```python
from build123d import *

# Parameters (mm, degrees)
BOSS_EXTRUDE1_DEPTH = 10
SKETCH2_W           = 90
SKETCH2_H           = 10
BOSS_EXTRUDE2_DEPTH = 13
SKETCH3_W           = 90
SKETCH3_H           = 10
BOSS_EXTRUDE3_DEPTH = 13
SKETCH4_R           = 3
CUT_EXTRUDE2_DEPTH  = 13


with BuildPart() as part:
    # Sketch1 → Boss-Extrude1 (new, symmetric)
    with BuildSketch(Plane.XY):
        Polygon((-49.027757444, 0), (100.972242556, 0), (-49.027757444, 13.123299529), align=None)
    extrude(amount=BOSS_EXTRUDE1_DEPTH, both=True)

    # Sketch2 → Boss-Extrude2 (add)
    with BuildSketch(Plane.XY.offset(10)):
        with Locations((30.972242556, 5)):
            Rectangle(SKETCH2_W, SKETCH2_H)
    extrude(amount=BOSS_EXTRUDE2_DEPTH)

    # Sketch3 → Boss-Extrude3 (add)
    with BuildSketch(Plane.XY.offset(-10)):
        with Locations((30.972242556, 5)):
            Rectangle(SKETCH3_W, SKETCH3_H)
    extrude(amount=-BOSS_EXTRUDE3_DEPTH)

    # Sketch4 → Cut-Extrude2 (cut)
    with BuildSketch(Plane.XZ.offset(-10)):
        with Locations(Location((-1.027757444, 16.5, 0), (0, 0, 180))):
            Circle(SKETCH4_R)
        with Locations(Location((62.972242556, 16.5, 0), (0, 0, 180))):
            Circle(SKETCH4_R)
        with Locations(Location((62.972242556, -16.5, 0), (0, 0, 180))):
            Circle(SKETCH4_R)
        with Locations(Location((-1.027757444, -16.5, 0), (0, 0, 180))):
            Circle(SKETCH4_R)
    extrude(amount=CUT_EXTRUDE2_DEPTH, mode=Mode.SUBTRACT)


solid = part.part
```
Here's how the part is built. I have some questions about the finished solid (model axes, mm). A direction names the side the tool comes from. Give positions to 0.01 mm unless a question says otherwise; leave off trailing zeros. Order: outer loops, then holes, each group sorted by start corner. A loop starts at its lowest first (then second) coordinate and runs counter-clockwise, first axis right, second up. Notation, with made-up numbers: M 13.25,-37.75 L 42.25,-37.75 A24 cw 42.25,-25.75 Z; hole C -9,42 d1. An arc over 180 degrees is marked long. Use a Markdown table: item, result. Add a question column.
1. If we mould it in two halves opening along Z, with no side actions, what happens to faces 5 (the flat face through (-14.028, 5, 16)), 6 (the cylindrical face through (60.2, 5.07, 17.65)), 7 (the flat face through (30, 5, 23))? For each: +Z half, -Z half, draft (parallel to the pull), parting line (faces both ways), or undercut.
2. I need wall thicknesses on probe 1 along X at (y, z) = (5.25, 16.5); probe 2 along Z at (x, y) = (-3.5, 9); probe 3 along Y at (x, z) = (16.5, -13). Which ranges of each line are inside material? Lowest first, please. Write a range as from..to.
3. Suppose I cut it at B-B (y = 8). List the corners of the cut face in (x, z) for me.
4. Suppose I cut it at D-D (x = 25.5). List the corners of the cut face in (y, z) for me.
5. Suppose I cut it at C-C (x = 0.5). List the corners of the cut face in (y, z) for me.
6. For pin 1 Ø2.5 at (x, y) = (88.5, 1.5) entering from -Z; pin 2 Ø5 at (x, y) = (-24, 3) entering from +Z; pin 3 Ø5 at (y, z) = (4.5, -15.5) entering from -X; pin 4 Ø5 at (x, z) = (-1.03, -16.5) entering from -Y, each with a flat end and sliding along its axis, tell me the tip position at first contact or that it passes through.
7. Suppose I cut it at A-A (z = 16.5). List the corners of the cut face in (x, y) for me.
8. On a 3-axis mill with a long thin cutter (end or side, diameter ignored), from which of +Z, -Z, +X, -X, +Y, -Y can I reach the whole of each face in a straight line? I mean faces 1 (the flat face through (75.972, 5, -16)), 2 (the flat face through (-14.028, 5, -16)), 3 (the flat face through (75.972, 5, 16)), 4 (the flat face through (27.02, 6.47, 0.14)). Say none if no direction works.
Results list:
| question | item | result |
|---|---|---|
| 1 | face 5 | draft |
| 1 | face 6 | undercut |
| 1 | face 7 | +Z half |
| 2 | probe 1 | x = -14.03..-4.03, 1.97..59.97, 65.97..75.97 |
| 2 | probe 2 | z = -23..-18.2, -14.8..14.8, 18.2..23 |
| 2 | probe 3 | y = 0..10 |
| 3 | outline | M -49.03,-10 L -14.03,-10 L -14.03,-23 L 75.97,-23 L 75.97,-10 L 9.53,-10 L 9.53,10 L 75.97,10 L 75.97,23 L -14.03,23 L -14.03,10 L -49.03,10 Z; hole C -1.03,-16.5 d6; hole C -1.03,16.5 d6; hole C 62.97,-16.5 d6; hole C 62.97,16.5 d6 |
| 4 | outline | M 0,-23 L 10,-23 L 10,-10 L 6.6,-10 L 6.6,10 L 10,10 L 10,23 L 0,23 Z |
| 5 | outline | M 0,-23 L 10,-23 L 10,-19.08 L 0,-19.08 Z; M 0,-13.92 L 10,-13.92 L 10,-10 L 8.79,-10 L 8.79,10 L 10,10 L 10,13.92 L 0,13.92 Z; M 0,19.08 L 10,19.08 L 10,23 L 0,23 Z |
| 6 | pin 1 | stops at z = -10 |
| 6 | pin 2 | stops at z = 10 |
| 6 | pin 3 | stops at x = -14.03 |
| 6 | pin 4 | passes through |
| 7 | outline | M -14.03,0 L -4.03,0 L -4.03,10 L -14.03,10 Z; M 1.97,0 L 59.97,0 L 59.97,10 L 1.97,10 Z; M 65.97,0 L 75.97,0 L 75.97,10 L 65.97,10 Z |
| 8 | face 1 | -Z, +X, +Y, -Y |
| 8 | face 2 | -Z, -X, +Y, -Y |
| 8 | face 3 | +Z, +X, +Y, -Y |
| 8 | face 4 | +X, +Y |
